```python
from build123d import *

# Parameters (mm, degrees)
SKETCH_1_R       = 1.25
BOARD_DEPTH      = 1
SKETCH_2_W       = 38
SKETCH_2_H       = 30
SCREEN_DEPTH     = 2
SCREEN_RADIUS_R  = 3.5
SKETCH_3_W       = 51
SKETCH_3_H       = 5
PLUG_DEPTH       = 7.5
SKETCH_4_W       = 15.14
SKETCH_4_H       = 20
SPEAKER_DEPTH    = 5
SKETCH_5_W       = 12.7
SKETCH_5_H       = 6
BUTTON_DEPTH     = 6
SKETCH_6_W       = 1
SKETCH_6_H       = 4
BUTTON_TAP_DEPTH = 1
SKETCH_7_W       = 1.5
SKETCH_7_H       = 1.5
RGB_LED_DEPTH    = 0.7
SKETCH_8_W       = 3.2
SKETCH_8_H       = 2.5
MIC_DEPTH        = 1.3
EXTRUDE_START    = 0.1
EXTRUDE_1_DEPTH  = 0.1


with BuildPart() as part:
    # 草图1 → board (new body)
    with BuildSketch(Plane(origin=(0, 0, 0), x_dir=(1, 0, 0), z_dir=(0, 1, 0))):
        with BuildLine():
            Line((-29.5, 15), (29.5, 15))
            ThreePointArc((29.5, 15), (31.621320344, 14.121320344), (32.5, 12))
            Line((32.5, 12), (32.5, -12))
            ThreePointArc((32.5, -12), (31.621320344, -14.121320344), (29.5, -15))
            Line((29.5, -15), (-29.5, -15))
            ThreePointArc((-29.5, -15), (-31.621320344, -14.121320344), (-32.5, -12))
            Line((-32.5, -12), (-32.5, 12))
            ThreePointArc((-32.5, 12), (-31.621320344, 14.121320344), (-29.5, 15))
        make_face()
        with Locations(Location((-29.5, 12, 0), (0, 0, 270))):
            Circle(SKETCH_1_R, mode=Mode.SUBTRACT)
        with Locations(Location((29.5, 12, 0), (0, 0, 270))):
            Circle(SKETCH_1_R, mode=Mode.SUBTRACT)
        with Locations(Location((-29.5, -12, 0), (0, 0, 270))):
            Circle(SKETCH_1_R, mode=Mode.SUBTRACT)
        with Locations(Location((29.5, -12, 0), (0, 0, 270))):
            Circle(SKETCH_1_R, mode=Mode.SUBTRACT)
    extrude(amount=BOARD_DEPTH)

    # 草图2 → screen (add)
    with BuildSketch(Plane(origin=(0, 1, 0), x_dir=(1, 0, 0), z_dir=(0, 1, 0))):
        with Locations((7.5, 0)):
            Rectangle(SKETCH_2_W, SKETCH_2_H)
    extrude(amount=SCREEN_DEPTH)

    # screen-radius
    screen_radius_edges = [part.edges().sort_by_distance(p)[0] for p in [
        (-11.5, 2, -15),
        (-11.5, 2, 15),
        (26.5, 2, 15),
        (26.5, 2, -15),
    ]]
    fillet(screen_radius_edges, radius=SCREEN_RADIUS_R)

    # 草图3 → plug (add)
    with BuildSketch(Plane.XZ):
        with Locations((0, -11.5)):
            Rectangle(SKETCH_3_W, SKETCH_3_H)
    extrude(amount=PLUG_DEPTH)

    # 草图4 → speaker (add)
    with BuildSketch(Plane.XZ):
        with Locations((-17.52, 2.68)):
            Rectangle(SKETCH_4_W, SKETCH_4_H)
    extrude(amount=SPEAKER_DEPTH)

    # 草图5 → button (add)
    with BuildSketch(Plane.XZ):
        with Locations((7.15, 12)):
            Rectangle(SKETCH_5_W, SKETCH_5_H)
    extrude(amount=BUTTON_DEPTH)

    # 草图6 → button-tap (add)
    with BuildSketch(Plane.XY.offset(15)):
        with Locations((9.5, -3)):
            Rectangle(SKETCH_6_W, SKETCH_6_H)
    extrude(amount=BUTTON_TAP_DEPTH)

    # 草图7 → rgb-led (add)
    with BuildSketch(Plane(origin=(0, 1, 0), x_dir=(1, 0, 0), z_dir=(0, 1, 0))):
        with Locations((29.25, 0)):
            Rectangle(SKETCH_7_W, SKETCH_7_H)
    extrude(amount=RGB_LED_DEPTH)

    # 草图8 → mic (add)
    with BuildSketch(Plane(origin=(0, 1, 0), x_dir=(1, 0, 0), z_dir=(0, 1, 0))):
        with Locations((-26.6, -0.25)):
            Rectangle(SKETCH_8_W, SKETCH_8_H)
    extrude(amount=MIC_DEPTH)

    # 草图9 → 凸台-拉伸1 (add)
    with BuildSketch(Plane(origin=(0, 3, 0), x_dir=(1, 0, 0), z_dir=(0, 1, 0)).offset(EXTRUDE_START)):
        with BuildLine():
            Line((26.5, -11.5), (26.5, 11.5))
            ThreePointArc((26.5, 11.5), (25.80624304, 13.591650066), (24, 14.854101966))
            Line((24, 14.854101966), (24, -14.854101966))
            ThreePointArc((24, -14.854101966), (25.80624304, -13.591650066), (26.5, -11.5))
        make_face()
    extrude(amount=-EXTRUDE_1_DEPTH)


solid = part.part
```
Here's how the part is built. I have some questions about the finished solid (model axes, mm). A direction names the side the tool comes from. Round coordinates to 2 decimals unless told otherwise and drop trailing zeros. Write each loop counter-clockwise with the first axis right and the second up, starting at its lowest first coordinate (ties: lowest second). Pieces come first, ordered by that corner, then holes.
Q1. If we section it at B-B on z = -5.5: Write out the boundary of the cut face in (x, y).
Q2. Will these pins go through, and if not, where does the flat tip stop? P1, Ø2, axis at x = -8.5, y = -3.5, coming from the +Z side; P2, Ø4, axis at x = -17.5, y = -3, coming from the -Z side; P3, Ø2, axis at x = 25, z = 10, coming from the -Y side.
Q3. If we section it at A-A on y = -3.75: Write out the boundary of the cut face in (x, z).
Q4. Please list where these lines run through material, in increasing order: probe 1 along X at (y, z) = (0.6, 12); probe 2 along Z at (x, y) = (20, -6.5); probe 3 along Y at (x, z) = (-11, 11.5).
Q5. If we section it at D-D on x = 11: Write out the boundary of the cut face in (y, z).
Q6. If we section it at C-C on x = -24: Write out the boundary of the cut face in (y, z).
Q7. If we mould it in two halves opening along Z, with no side actions, what happens to faces 4 (the cylindrical face through (31.64, 0.49, 14.1)), 5 (the flat face through (0, -4, -14)), 6 (the flat face through (25.5, -4, -12)), 7 (the cylindrical face through (-28.655, 0.493, 11.079))? For each: +Z half, -Z half, draft (parallel to the pull), parting line (faces both ways), or undercut.
Q8. Which directions (+Z, -Z, +X, -X, +Y, -Y) give clear straight access to the entire face, cutting with the end or side of a thin tool? Please do faces 1 (the cylindrical face through (-10.45, 2.01, -14)), 2 (the flat face through (-25.09, -2, 3)), 3 (the flat face through (0.8, -3, 12)).
Answer below:
1. outline: (-32.5, 0) - (-25.09, 0) - (-25.09, -5) - (-9.95, -5) - (-9.95, 0) - (32.5, 0) - (32.5, 1) - (26.5, 1) - (26.5, 3.1) - (24, 3.1) - (24, 3) - (-11.5, 3) - (-11.5, 1) - (-32.5, 1) - close
2. P1: stops at z = -9
2. P2: stops at z = -14
2. P3: stops at y = 0
3. outline: (-25.5, -14) - (25.5, -14) - (25.5, -9) - (-25.5, -9) - close; (-25.09, -7.32) - (-9.95, -7.32) - (-9.95, 12.68) - (-25.09, 12.68) - close; (0.8, 9) - (13.5, 9) - (13.5, 15) - (10, 15) - (10, 16) - (9, 16) - (9, 15) - (0.8, 15) - close
4. probe 1: x = -32.5 to -30.75, -28.25 to 28.25, 30.75 to 32.5
4. probe 2: z = -14 to -9
4. probe 3: y = -5 to 3
5. outline: (-7.5, -14) - (0, -14) - (0, -15) - (3, -15) - (3, 15) - (-6, 15) - (-6, 9) - (0, 9) - (0, -9) - (-7.5, -9) - close
6. outline: (-7.5, -14) - (0, -14) - (0, -15) - (1, -15) - (1, 15) - (0, 15) - (0, 12.68) - (-5, 12.68) - (-5, -7.32) - (0, -7.32) - (0, -9) - (-7.5, -9) - close
7. face 4: +Z half
7. face 5: -Z half
7. face 6: draft
7. face 7: undercut
8. face 1: -Z, -X, +Y
8. face 2: +Z, -X, -Y
8. face 3: +Z, -Y
